Geometry check sheet. Reference: the model listing, model coordinates, mm. Face numbers are marked on the shaded views. Round coordinates to 2 decimals unless told otherwise and drop trailing zeros. Order: outer loops, then holes, each group sorted by start corner. A loop starts at its lowest first (then second) coordinate and runs counter-clockwise, first axis right, second up. Notation, with made-up numbers: (59, 69.5) -> (81, 69.5) arc R30 ccw to (81, 100.5) -> close; hole circle Ø2 at (63, 11). An arc over 180 degrees is marked (long way). Use a Markdown table: item, result. Add a question column.
Item 1: Gauge pin test, flat ends, axial feed: pin 1 Ø1.4 at (x, y) = (-40.5, -6) entering from -Z; pin 2 Ø1.5 at (x, y) = (31, 24) entering from -Z; pin 3 Ø2 at (x, z) = (-40, 20.5) entering from +Y. Record the tip position at first contact, or that the pin passes through.
Item 2: Sectioned sample at B-B, the plane z = 0. Record the cut outline in (x, y).
Item 3: Material ranges on probe 1 along Y at (x, z) = (24.5, -41); probe 2 along Y at (x, z) = (-7, 44); probe 3 along X at (y, z) = (13, -18), recorded low to high. Write a range as [from, to].
Item 4: Sectioned sample at D-D, the plane x = 35.5. Record the cut outline in (y, z).
Item 5: Mould release check, pull along Y, two halves, no side actions. Record for the marked faces 1, 2 and 3: pulls with the +Y half, pulls with the -Y half, needs draft (parallel to the pull), parting line crosses it, or undercut.
Item 6: Sectioned sample at A-A, the plane x = 0. Record the cut outline in (y, z), and give its area (3 significant figures).
Item 7: Sectioned sample at C-C, the plane z = -35. Record the cut outline in (x, y), and give its area (3 significant figures).
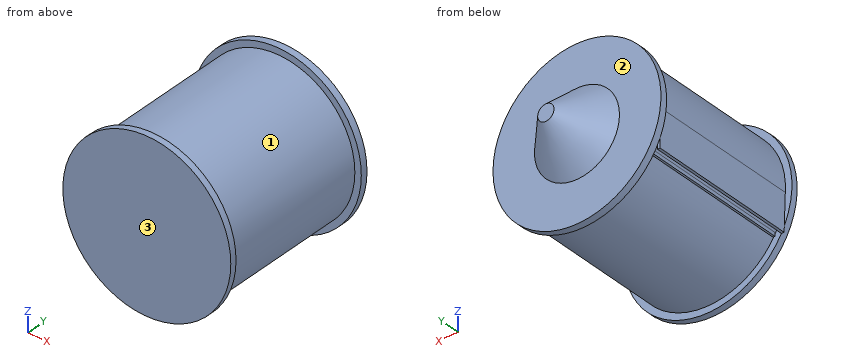
from build123d import *

# Parameters (mm, degrees)
CROQUIS3_W              = 2.5
CROQUIS3_H              = 93.200468797
CROQUIS3_H_2            = 93.221326365
SALIENTE_EXTRUIR1_DEPTH = 25
SALIENTE_EXTRUIR1_TAPER = 1


with BuildPart() as part:
    # Croquis1 → Revolución1 (revolve)
    with BuildSketch(Plane.XY):
        Polygon((0, 38.800633525), (0, -62.573128225), (50.821461866, -62.573128225), (50.821461866, -58.674137389), (46.92247103, -58.674137389), (46.92247103, 34.547188976), (50.821461866, 34.547188976), (50.821461866, 38.800633525), align=None)
    revolve(axis=Axis((0, 38.800633525, 0), (0, -1, 0)))

    # Croquis3 → Saliente-Extruir1 (add)
    with BuildSketch(Plane.XY):
        with Locations((-45.646866178, -12.07390299)):
            Rectangle(CROQUIS3_W, CROQUIS3_H)
        with Locations((-40.124494984, -12.063474207)):
            Rectangle(CROQUIS3_W, CROQUIS3_H_2)
    extrude(amount=-SALIENTE_EXTRUIR1_DEPTH, taper=SALIENTE_EXTRUIR1_TAPER)

    # Croquis6 → Revolución2 (revolve)
    with BuildSketch(Plane.XY):
        Polygon((0, 61.973262814), (0, 34.547188976), (-30.940786447, 34.547188976), (-30.940786447, 38.800633525), (-25.72291089, 38.800633525), (-4.924695463, 61.973262814), align=None)
    revolve(axis=Axis((0, 61.973262814, 0), (0, -1, 0)))


solid = part.part
Found:
| question | item | result |
|---|---|---|
| 1 | pin 1 | stops at z = -25 |
| 1 | pin 2 | stops at z = -35.87 |
| 1 | pin 3 | stops at y = 38.8 |
| 2 | outline | (-50.82, -62.57) -> (50.82, -62.57) -> (50.82, -58.67) -> (46.92, -58.67) -> (46.92, 34.55) -> (50.82, 34.55) -> (50.82, 38.8) -> (25.72, 38.8) -> (4.92, 61.97) -> (-4.92, 61.97) -> (-25.72, 38.8) -> (-50.82, 38.8) -> (-50.82, 34.55) -> (-46.92, 34.55) -> (-46.92, -58.67) -> (-50.82, -58.67) -> close |
| 3 | probe 1 | y = [-62.57, -58.67], [34.55, 38.8] |
| 3 | probe 2 | y = [-62.57, 38.8] |
| 3 | probe 3 | x = [-46.58, -44.71], [-43.33, 43.33] |
| 4 | outline | (-62.57, -36.37) -> (-58.67, -36.37) -> (-58.67, -30.68) -> (34.55, -30.68) -> (34.55, -36.37) -> (38.8, -36.37) -> (38.8, 36.37) -> (34.55, 36.37) -> (34.55, 30.68) -> (-58.67, 30.68) -> (-58.67, 36.37) -> (-62.57, 36.37) -> close |
| 5 | face 1 | undercut |
| 5 | face 2 | pulls with the +Y half |
| 5 | face 3 | pulls with the -Y half |
| 6 | outline | (-62.57, -50.82) -> (-58.67, -50.82) -> (-58.67, -46.92) -> (34.55, -46.92) -> (34.55, -50.82) -> (38.8, -50.82) -> (38.8, -25.72) -> (61.97, -4.92) -> (61.97, 4.92) -> (38.8, 25.72) -> (38.8, 50.82) -> (34.55, 50.82) -> (34.55, 46.92) -> (-58.67, 46.92) -> (-58.67, 50.82) -> (-62.57, 50.82) -> close |
| 6 | area | 10,300 mm2 |
| 7 | outline | (-36.85, -62.57) -> (36.85, -62.57) -> (36.85, -58.67) -> (31.25, -58.67) -> (31.25, 34.55) -> (36.85, 34.55) -> (36.85, 38.8) -> (-36.85, 38.8) -> (-36.85, 34.55) -> (-31.25, 34.55) -> (-31.25, -58.67) -> (-36.85, -58.67) -> close |
| 7 | area | 6,430 mm2 |
